The listing builds one solid part. Answer for the finished solid, in the listing's coordinates (mm). Face numbers are marked on the shaded views. A direction names the side the tool comes from. Round coordinates to 2 decimals unless told otherwise and drop trailing zeros. Order: outer loops, then holes, each group sorted by start corner. A loop starts at its lowest first (then second) coordinate and runs counter-clockwise, first axis right, second up. Notation, with made-up numbers: (37, -30) -> (70, -30) arc R21 ccw to (70, 2) -> close; hole circle Ø7 at (44, -23.75). An arc over 180 degrees is marked (long way). Answer in a Markdown table with one row per item. Add a question column.
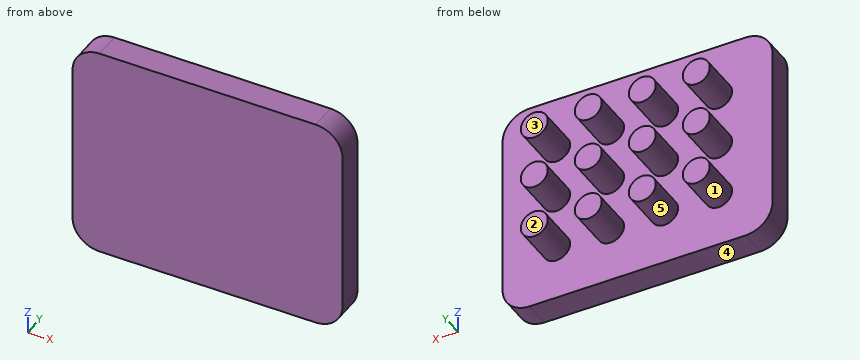
Autodesk Inventor part; units mm, degrees
ref_plane "YZ Plane" through (0, 0, 0) normal (1, 0, 0) x (0, 1, 0)
ref_plane "XZ Plane" through (0, 0, 0) normal (0, 1, 0) x (-1, 0, 0)
ref_plane "XY Plane" through (0, 0, 0) normal (0, 0, 1) x (1, 0, 0)
sketch "草圖1" plane through (0, 0, 0) normal (0, 1, 0) x (-1, 0, 0)
  line L0 (-10, 0) -> (-90, 0)
  line L1 (-100, -10) -> (-100, -70)
  line L2 (-90, -80) -> (-10, -80)
  line L3 (0, -70) -> (0, -10)
  arc A0 (-90, 0) -> (-100, -10) centre (-90, -10) ccw
  arc A1 (-100, -70) -> (-90, -80) centre (-90, -70) ccw
  arc A2 (-10, -80) -> (0, -70) centre (-10, -70) ccw
  arc A3 (0, -10) -> (-10, 0) centre (-10, -10) ccw
  point P0 (0, 0)
  point P1 (-100, 0)
  point P2 (0, -80)
  dimension "d0" = 100
  dimension "d1" = 80
  dimension "d2" = 10
extrude "擠出1" add sketch "草圖1" along normal blind 10
sketch "草圖2" plane through (0, 10, 0) normal (0, 1, 0) x (1, 0, 0)
  circle A0 centre (80, 20) radius 5
  line L0 (100, 10) -> (100, 70)
  line L1 (10, 0) -> (90, 0)
  point P0 (0, 0)
  dimension "d5" = 20
  dimension "d6" = 20
  dimension "d7" = 10
extrude "擠出2" add sketch "草圖2" along normal blind 15
pattern_linear "矩形陣列1" count 4 spacing 20 along (-1, 0, 0) count 3 spacing 20 along (0, 0, -1) of "擠出2"
properties part number "練習二"
1. For the marked faces 1 and 2, determine the directions among +Z, -Z, +X, -X, +Y, -Y from which every point of the face is accessible in a straight line to the end or side of a thin tool.
2. Each of these flat-tipped pins is pushed along its axis until it touches: pin 1 (5 mm diameter, centred on x = 31, z = -8.5, fed in from +Y); pin 2 (1.5 mm diameter, centred on x = 44.5, y = 18.5, fed in from -Z); pin 3 (5 mm diameter, centred on y = 14.5, z = -67, fed in from -X). Where does it stop, or does it pass through?
3. The mould has two halves that part along Z. Classify the marked faces 3, 4 and 5: released by +Z, released by -Z, zero draft, split by the parting line, or undercut.
4. The part is cut by section D-D (z = -28.5). Give the vertices of the cut face in (x, y).
5. The part is cut by section C-C (z = -20). Give the vertices of the cut face in (x, y), then the cut area to 3 significant figures.
6. The part is cut by section A-A (y = 19.25). Give the number of separate pieces and of enclosed holes in the cut face, then the cut area to 3 significant figures.
7. The part is cut by section B-B (x = 80). Give the vertices of the cut face in (y, z).
8. Straight lines are drawn through the part: line 1 along X through (y, z) = (18.25, -60.5); line 2 along Z through (x, y) = (79.5, 14.5); line 3 along X through (y, z) = (16, -58.5). For each, find the intervals that lie inside material, in ascending order.
Report:
| question | item | result |
|---|---|---|
| 1 | face 1 | +Y |
| 1 | face 2 | +Z, -Z, +X, -X, +Y |
| 2 | pin 1 | stops at y = 10 |
| 2 | pin 2 | stops at z = -63.31 |
| 2 | pin 3 | stops at x = 17.82 |
| 3 | face 3 | zero draft |
| 3 | face 4 | released by -Z |
| 3 | face 5 | undercut |
| 4 | outline | (0, 0) -> (100, 0) -> (100, 10) -> (0, 10) -> close |
| 5 | outline | (0, 0) -> (100, 0) -> (100, 10) -> (85, 10) -> (85, 25) -> (75, 25) -> (75, 10) -> (65, 10) -> (65, 25) -> (55, 25) -> (55, 10) -> (45, 10) -> (45, 25) -> (35, 25) -> (35, 10) -> (25, 10) -> (25, 25) -> (15, 25) -> (15, 10) -> (0, 10) -> close |
| 5 | area | 1,600 mm^2 |
| 6 | separate pieces | 12 |
| 6 | enclosed holes | 0 |
| 6 | area | 942 mm^2 |
| 7 | outline | (0, -80) -> (10, -80) -> (10, -65) -> (25, -65) -> (25, -55) -> (10, -55) -> (10, -45) -> (25, -45) -> (25, -35) -> (10, -35) -> (10, -25) -> (25, -25) -> (25, -15) -> (10, -15) -> (10, 0) -> (0, 0) -> close |
| 8 | line 1 | x = 15.03 to 24.97, 35.03 to 44.97, 55.03 to 64.97, 75.03 to 84.97 |
| 8 | line 2 | z = -64.97 to -55.03, -44.97 to -35.03, -24.97 to -15.03 |
| 8 | line 3 | x = 15.23 to 24.77, 35.23 to 44.77, 55.23 to 64.77, 75.23 to 84.77 |
